Source: CAD feature listing. Evaluate the final solid. Frame: model axes, mm. Face numbers are marked on the shaded views. A direction names the side the tool comes from. Give positions to 0.01 mm unless a question says otherwise; leave off trailing zeros. Write each loop counter-clockwise with the first axis right and the second up, starting at its lowest first coordinate (ties: lowest second). Pieces come first, ordered by that corner, then holes. Notation, with made-up numbers: M 39.5,16.5 L 51.5,16.5 A27 ccw 51.5,51.5 Z; hole C -37.5,89 d4. An arc over 180 degrees is marked long. Return JSON: item names as keys, results as strings.
```python
from build123d import *


with BuildPart() as f1:
    # F0 (on Front) → F1 (revolve)
    with BuildSketch(Plane.XZ):
        Polygon((11.832037, -1.892192), (11.832037, 3.574136), (8.841912, 1.892188), align=None)
        Polygon((26.385557, 48.566248), (14.822163, 42.258941), (14.822163, 35.320906), align=None)
        Polygon((34.795295, 34.269687), (14.822163, 29.223844), (14.822163, 24.59849), align=None)
        Polygon((11.832037, 3.574136), (8.841912, 5.256084), (8.841912, 1.892188), align=None)
        Polygon((14.822163, 42.258941), (14.822163, 55.924769), (8.841912, 54.663308), (8.841912, 5.256084), (11.832037, 3.574136), (14.822163, 1.892188), (16.714357, 5.256084), (39.000165, 14.717042), (14.822163, 14.717042), (14.822163, 24.59849), (14.822163, 29.223844), (14.822163, 35.320906), align=None)
    revolve(axis=Axis((8.841912, 0, 29.959696), (0, 0, 1)))


solid = f1.part
```
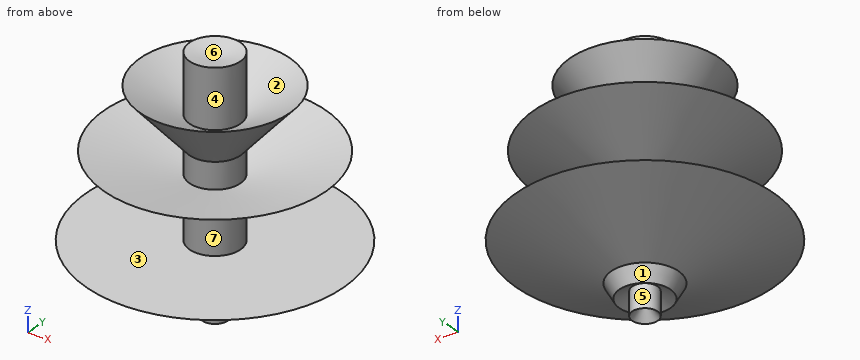
1) Draft query along Y for the marked faces 1, 2, 3 and 4. Return one class per face: released by +Y, released by -Y, zero draft, split by the parting line, or undercut.
Numbers:
{"face 1": "split by the parting line", "face 2": "undercut", "face 3": "zero draft", "face 4": "undercut"}
2) Set-up query: the marked faces 5, 6 and 7. Return all of +Z, -Z, +X, -X, +Y, -Y with unobstructed straight access to the full face (end or side cutting, diameter ignored); none if empty.
Numbers:
{"face 5": "-Z", "face 6": "+Z", "face 7": "none"}
3) Line query: line 1 (Z direction, x = 11, y = -9); line 2 (X direction, y = -0.5, z = 44.5); line 3 (Y direction, x = 4, z = 47). Output: solid intervals per line, ascending. Write a range as [from, to].
Numbers:
{"line 1": "z = [5.84, 14.72], [26.18, 30.05], [39.07, 44.05]", "line 2": "x = [-5.14, -1.23], [2.88, 14.8], [18.92, 22.83]", "line 3": "y = [-15.43, -13.85], [-3.51, 3.51], [13.85, 15.43]"}
4) Contact query for flat-ended pins moving along their axis: pin 1 Ø8 at (x, y) = (18.5, 17.5) entering from +Z; pin 2 Ø3 at (y, z) = (-5.5, 47.5) entering from -X; pin 3 Ø3 at (x, z) = (2, 22) entering from -Y. Output: stop coordinate, or through.
Numbers:
{"pin 1": "stops at z = 48.57", "pin 2": "stops at x = -8.13", "pin 3": "stops at y = -2.69"}
5) Cut plane A-A, the plane z = 46. Return the cut outline in (x, y), then the cut area to 3 significant figures.
Numbers:
{"outline": "C 8.84,0 d30.61; C 8.84,0 d11.96; hole C 8.84,0 d25.68", "area": "330 mm²"}
6) Cut plane B-B, the plane x = 23. Give the number of separate pieces and of enclosed holes in the cut face, then the cut area to 3 significant figures.
Numbers:
{"separate pieces": "3", "enclosed holes": "0", "area": "325 mm²"}
7) Cut plane C-C, the plane z = 19. Return the cut outline in (x, y), then the cut area to 3 significant figures.
Numbers:
{"outline": "C 8.84,0 d11.96", "area": "112 mm²"}
